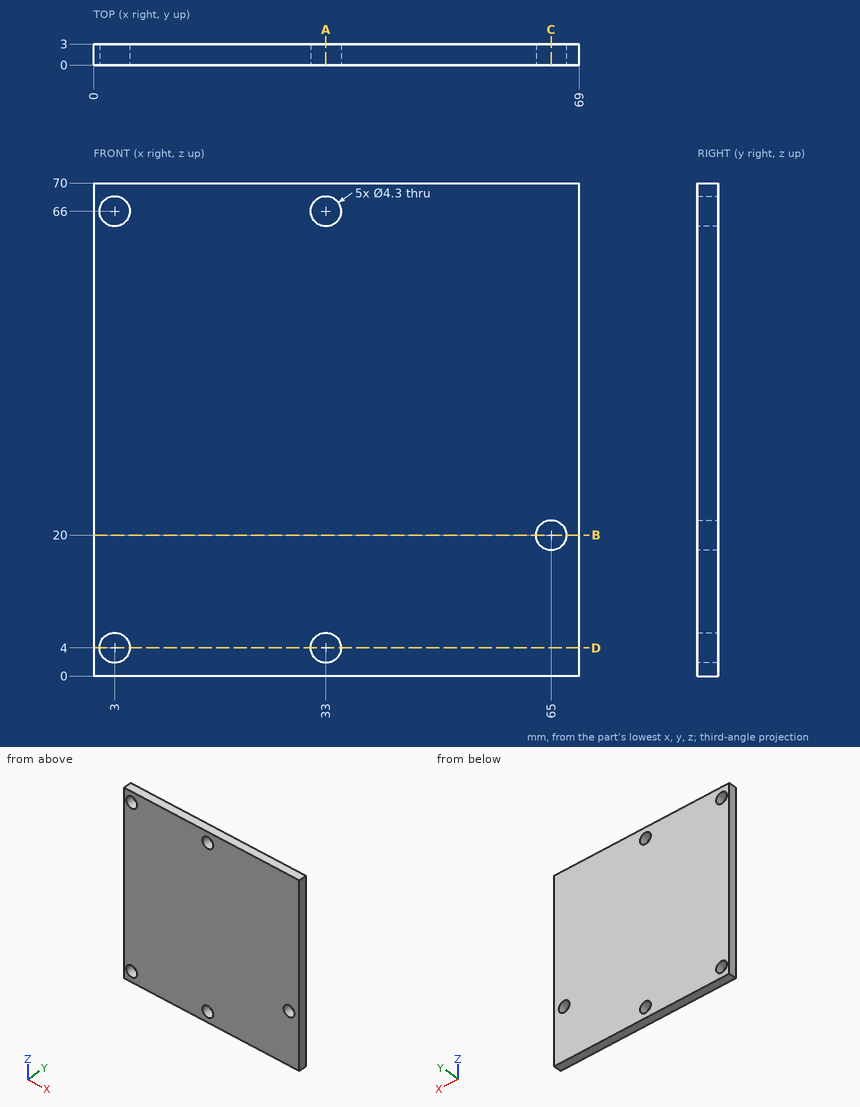
Geometry: see drawing. Coordinates: mm, zero at the bounding-box minimum. Give positions to 0.01 mm unless a question says otherwise; leave off trailing zeros. Loops run counter-clockwise (first coordinate to the right, second up) from the corner with the lowest first, then second, coordinate; pieces in that order, holes last. Notation, with made-up numbers: (1.25, 46) -> (25.25, 46) arc R6 ccw to (25.25, 51) -> close; hole circle Ø1 at (57, -12.5). An arc over 180 degrees is marked (long way). Use one line per item in the form item = value.
Item 1: Section query A-A on x = 33. Output: boundary loops of the cut face in (y, z), and give its area (3 significant figures).
A:
outline = (0, 0) -> (3, 0) -> (3, 1.85) -> (0, 1.85) -> close; (0, 6.15) -> (3, 6.15) -> (3, 63.85) -> (0, 63.85) -> close; (0, 68.15) -> (3, 68.15) -> (3, 70) -> (0, 70) -> close
area = 184 mm^2
Item 2: Pin query (flat end, axial travel): P1, Ø4, axis at x = 3, z = 4, coming from the -Y side; P2, Ø7, axis at x = 33, z = 4, coming from the -Y side. Return the tip coordinate at first contact, or that it passes through.
A:
P1 = through
P2 = 0
Item 3: Line query: probe 1 along X at (y, z) = (2.05, 66); probe 2 along Z at (x, y) = (34, 2.4). Output: solid intervals per line, ascending.
A:
probe_1 = 0 to 0.85, 5.15 to 30.85, 35.15 to 69
probe_2 = 0 to 2.1, 5.9 to 64.1, 67.9 to 70
Item 4: Section query C-C on x = 65. Output: boundary loops of the cut face in (y, z), and give its area (3 significant figures).
A:
outline = (0, 0) -> (3, 0) -> (3, 17.85) -> (0, 17.85) -> close; (0, 22.15) -> (3, 22.15) -> (3, 70) -> (0, 70) -> close
area = 197 mm^2
Item 5: Section query D-D on z = 4. Output: boundary loops of the cut face in (x, y).
A:
outline = (0, 0) -> (0.85, 0) -> (0.85, 3) -> (0, 3) -> close; (5.15, 0) -> (30.85, 0) -> (30.85, 3) -> (5.15, 3) -> close; (35.15, 0) -> (69, 0) -> (69, 3) -> (35.15, 3) -> close
Item 6: Section query B-B on z = 20. Output: boundary loops of the cut face in (x, y).
A:
outline = (0, 0) -> (62.85, 0) -> (62.85, 3) -> (0, 3) -> close; (67.15, 0) -> (69, 0) -> (69, 3) -> (67.15, 3) -> close
